Source: CAD feature listing. Evaluate the final solid. Frame: model axes, mm. A direction names the side the tool comes from. Give positions to 0.01 mm unless a question says otherwise; leave off trailing zeros. Loops run counter-clockwise (first coordinate to the right, second up) from the corner with the lowest first, then second, coordinate; pieces in that order, holes last. Notation, with made-up numbers: M 63.5,88.25 L 103.5,88.25 A13 ccw 103.5,107.25 Z; hole C -13,41.5 d4. An arc over 180 degrees is marked long. Answer in a Markdown table with one row per item.
```python
from build123d import *

# Parameters (mm, degrees)
SKETCH1_R           = 6
BOSS_EXTRUDE1_DEPTH = 24
SKETCH2_R           = 8.5
BOSS_EXTRUDE2_DEPTH = 7
BOSS_EXTRUDE2_TAPER = 10
BOSS_EXTRUDE3_START = -7
SKETCH3_R           = 6
BOSS_EXTRUDE3_DEPTH = 4


with BuildPart() as part:
    # Sketch1 → Boss-Extrude1 (new body)
    with BuildSketch(Plane.XY):
        Circle(SKETCH1_R)
    extrude(amount=BOSS_EXTRUDE1_DEPTH)

    # Sketch2 → Boss-Extrude2 (add)
    with BuildSketch(Plane.XY):
        Circle(SKETCH2_R)
    extrude(amount=-BOSS_EXTRUDE2_DEPTH, taper=BOSS_EXTRUDE2_TAPER)

    # Sketch3 → Boss-Extrude3 (add)
    with BuildSketch(Plane.XY.offset(BOSS_EXTRUDE3_START)):
        Circle(SKETCH3_R)
    extrude(amount=-BOSS_EXTRUDE3_DEPTH)


solid = part.part
```
Q1. Reachability of faces 1 (the cylindrical face through (-6, 0, -9)), 2 (the flat face through (2, 6, 0)), 3 (the flat face through (0, 0, 24)) from +Z, -Z, +X, -X, +Y, -Y: full face, straight path, thin tool, end or side. Return the list, or none.
Values follow:
| item | result |
|---|---|
| face 1 | -Z |
| face 2 | +Z |
| face 3 | +Z, +X, -X, +Y, -Y |
Q2. Section query B-B (z = 9). Output: boundary loops of the cut face in (x, y), plus the area to 3 significant figures.
Values follow:
| item | result |
|---|---|
| outline | C 0,0 d12 |
| area | 113 mm^2 |
Q3. Contact query for flat-ended pins moving along their axis: pin 1 Ø3 at (x, z) = (3.5, 6) entering from +Y; pin 2 Ø2 at (x, z) = (6, -1) entering from +Y; pin 3 Ø6 at (x, z) = (0, 19.5) entering from +Y. Output: stop coordinate, or through.
Values follow:
| item | result |
|---|---|
| pin 1 | y = 5.66 |
| pin 2 | y = 6.69 |
| pin 3 | y = 6 |
Q4. Ray query, probe 1 along Z at (x, y) = (-6, 2.5); probe 2 along X at (y, z) = (-5, 20.5); probe 3 along Y at (x, z) = (1.5, 22.5). Return the intervals inside material, ascending. Write a range as from..to.
Values follow:
| item | result |
|---|---|
| probe 1 | -7..0 |
| probe 2 | -3.32..3.32 |
| probe 3 | -5.81..5.81 |
Q5. Section query C-C (z = -5). Output: boundary loops of the cut face in (x, y), plus the area to 3 significant figures.
Values follow:
| item | result |
|---|---|
| outline | C 0,0 d15.24 |
| area | 182 mm^2 |
Q6. Section query A-A (x = 0). Output: boundary loops of the cut face in (y, z), plus the area to 3 significant figures.
Values follow:
| item | result |
|---|---|
| outline | M -8.5,0 L -7.27,-7 L -6,-7 L -6,-11 L 6,-11 L 6,-7 L 7.27,-7 L 8.5,0 L 6,0 L 6,24 L -6,24 L -6,0 Z |
| area | 446 mm^2 |
